Verification items for the finished model (mm, model axes). Face numbers are marked on the shaded views. A direction names the side the tool comes from. Round coordinates to 2 decimals unless told otherwise and drop trailing zeros. Write each loop counter-clockwise with the first axis right and the second up, starting at its lowest first coordinate (ties: lowest second). Pieces come first, ordered by that corner, then holes. Notation, with made-up numbers: M 37,84.25 L 48,84.25 A22 ccw 48,99.25 Z; hole C -13,68 d3. An arc over 180 degrees is marked long. Use a Markdown table: item, result. Add a question column.
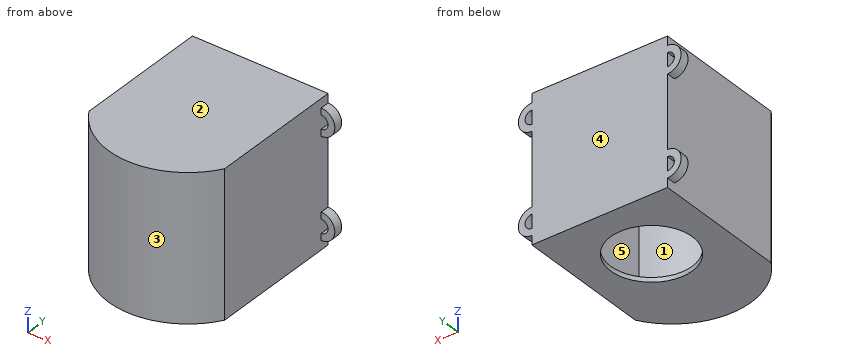
from build123d import *

# Parameters (mm, degrees)
F0_R     = 45
F1_DEPTH = 160
F2_T     = -5
F3_DEPTH = 5
F5_DEPTH = 10


with BuildPart() as f1:
    # F0 (on Top) → F1 (new body)
    with BuildSketch(Plane.XY):
        with BuildLine():
            Line((75, -75), (75, 75))
            Line((75, 75), (-75, 75))
            Line((-75, 75), (-75, -75))
            ThreePointArc((-75, -75), (0, -117.319724), (75, -75))
        make_face()
        Circle(F0_R, mode=Mode.SUBTRACT)
        Circle(F0_R)
    extrude(amount=F1_DEPTH)

    # F2
    f2_openings = [f1.faces().sort_by_distance(p)[0] for p in [
        (0, -15.361785, 0),
    ]]
    offset(amount=F2_T, openings=f2_openings)

    # F0 (on Top) → F3 (join)
    with BuildSketch(Plane.XY):
        with BuildLine():
            Line((75, -75), (75, 75))
            Line((75, 75), (-75, 75))
            Line((-75, 75), (-75, -75))
            ThreePointArc((-75, -75), (0, -117.319724), (75, -75))
        make_face()
        Circle(F0_R, mode=Mode.SUBTRACT)
    extrude(amount=F3_DEPTH)

    # F4 (on face) → F5 (join)
    with BuildSketch(Plane(origin=(0, 75, 0), x_dir=(-1, 0, 0), z_dir=(0, 1, 0))):
        with BuildLine():
            ThreePointArc((-75, 150), (-90, 135), (-75, 120))
            Line((-75, 120), (-75, 127.5))
            ThreePointArc((-75, 127.5), (-82.5, 135), (-75, 142.5))
            Line((-75, 142.5), (-75, 150))
        make_face()
        with BuildLine():
            Line((75, 127.5), (75, 120))
            ThreePointArc((75, 120), (90, 135), (75, 150))
            Line((75, 150), (75, 142.5))
            ThreePointArc((75, 142.5), (82.5, 135), (75, 127.5))
        make_face()
        with BuildLine():
            ThreePointArc((-75, 40), (-90, 25), (-75, 10))
            Line((-75, 10), (-75, 17.5))
            ThreePointArc((-75, 17.5), (-82.5, 25), (-75, 32.5))
            Line((-75, 32.5), (-75, 40))
        make_face()
        with BuildLine():
            Line((75, 17.5), (75, 10))
            ThreePointArc((75, 10), (90, 25), (75, 40))
            Line((75, 40), (75, 32.5))
            ThreePointArc((75, 32.5), (82.5, 25), (75, 17.5))
        make_face()
    extrude(amount=-F5_DEPTH)


solid = f1.part
1. Cross-section at B-B on y = -64. Enter the section's corners in (x, z), plus the area to 3 significant figures.
2. Cross-section at A-A on z = 25. Enter the section's corners in (x, y), plus the area to 3 significant figures.
3. Scan lines: line 1 along Y through (x, z) = (0, 3); line 2 along X through (y, z) = (-20.5, 53); line 3 along Z through (x, y) = (54.5, -64.5). Record each from-to range of solid material in increasing order. Write a range as from..to.
4. Access from +Z, -Z, +X, -X, +Y, -Y to the whole of each face (thin tool, end or side, straight path). Record for the marked faces 4 and 5.
5. Cross-section at C-C on x = -67. Enter the section's corners in (y, z).
6. Cross-section at D-D on y = 0. Enter the section's corners in (x, z), plus the area to 3 significant figures.
7. Depth check by flat-ended pin: pin 1 Ø4.5 at (x, z) = (85.5, 134.5) entering from -Y; pin 2 Ø1.5 at (y, z) = (-46.5, 92.5) entering from -X; pin 3 Ø1.5 at (x, z) = (37.5, 78.5) entering from -Y. Enter the tip coordinate at first touch or a pass-through.
8. Release check for a two-part mould opening along Z. For the marked faces 1, 2 and 3 record: +Z half, -Z half, draft (parallel to the pull), parting line (faces both ways), or undercut.
Answer:
| question | item | result |
|---|---|---|
| 1 | outline | M -75,0 L 75,0 L 75,160 L -75,160 Z; hole M -70,5 L 70,5 L 70,155 L -70,155 Z |
| 1 | area | 3,000 mm^2 |
| 2 | outline | M -90,65 L -82.5,65 L -82.5,75 L -90,75 Z; M -75,-75 A87.62 ccw 75,-75 L 75,75 L -75,75 Z; M 82.5,65 L 90,65 L 90,75 L 82.5,75 Z; hole M -70,-73.59 A82.62 ccw 70,-73.59 L 70,70 L -70,70 Z |
| 2 | area | 3,210 mm^2 |
| 3 | line 1 | y = -117.32..-45, 45..75 |
| 3 | line 2 | x = -75..-70, 70..75 |
| 3 | line 3 | z = 0..5, 155..160 |
| 4 | face 4 | +Z, -Z, +X, -X, +Y |
| 4 | face 5 | none |
| 5 | outline | M -86.16,0 L 75,0 L 75,160 L -86.16,160 Z; hole M -78.04,5 L 70,5 L 70,155 L -78.04,155 Z |
| 6 | outline | M -75,0 L -45,0 L -45,5 L -70,5 L -70,155 L 70,155 L 70,5 L 45,5 L 45,0 L 75,0 L 75,160 L -75,160 Z |
| 6 | area | 2,550 mm^2 |
| 7 | pin 1 | stops at y = 65 |
| 7 | pin 2 | stops at x = -75 |
| 7 | pin 3 | stops at y = -109.24 |
| 8 | face 1 | undercut |
| 8 | face 2 | +Z half |
| 8 | face 3 | draft |
